Here's how the part is built. I have some questions about the finished solid (model axes, mm). A direction names the side the tool comes from. Round coordinates to 2 decimals unless told otherwise and drop trailing zeros. Loops run counter-clockwise (first coordinate to the right, second up) from the corner with the lowest first, then second, coordinate; pieces in that order, holes last. Notation, with made-up numbers: M -19.5,14.25 L 5.5,14.25 A27 ccw 5.5,38.25 Z; hole C -0.5,-40 d5. An arc over 180 degrees is marked long. Put each result on its own line as item: value. Start each with the question number.
```python
from build123d import *

# Parameters (mm, degrees)
SKETCH_1_W          = 17.5
SKETCH_1_H          = 17.5
EXTRUDE_1_DEPTH     = 8
SKETCH_2_R          = 1.35
CUT_EXTRUDE_1_DEPTH = 22.137939824
CUT_EXTRUDE_2_DEPTH = 4
SKETCH_5_W          = 6.75
SKETCH_5_H          = 17.5
EXTRUDE_3_DEPTH     = 0.2
SKETCH_6_W          = 9.75
SKETCH_6_H          = 22
EXTRUDE_4_DEPTH     = 2.5


with BuildPart() as part:
    # 草图1 → 凸台-拉伸1 (new body)
    with BuildSketch(Plane(origin=(0, 0, 0), x_dir=(1, 0, 0), z_dir=(0, 1, 0))):
        Rectangle(SKETCH_1_W, SKETCH_1_H)
    extrude(amount=EXTRUDE_1_DEPTH)

    # 草图2 → 切除-拉伸1 (cut, through all)
    with BuildSketch(Plane(origin=(8.75, 0, 0), x_dir=(0, 0, -1), z_dir=(1, 0, 0))):
        with Locations((5, 4)):
            Circle(SKETCH_2_R)
        with Locations(Location((-5, 4, 0), (0, 0, 180))):
            Circle(SKETCH_2_R)
    extrude(amount=-CUT_EXTRUDE_1_DEPTH, mode=Mode.SUBTRACT)

    # 草图3 → 切除-拉伸2 (cut)
    with BuildSketch(Plane(origin=(8.75, 0, 0), x_dir=(0, 0, -1), z_dir=(1, 0, 0))):
        Polygon((7.886751346, 4), (6.443375673, 6.5), (3.556624327, 6.5), (2.113248654, 4), (3.556624327, 1.5), (6.443375673, 1.5), align=None)
        Polygon((-6.443375673, 1.5), (-7.886751346, 4), (-6.443375673, 6.5), (-3.556624327, 6.5), (-2.113248654, 4), (-3.556624327, 1.5), align=None)
    extrude(amount=-CUT_EXTRUDE_2_DEPTH, mode=Mode.SUBTRACT)

    # 草图5 → 凸台-拉伸3 (add)
    with BuildSketch(Plane.XZ):
        with Locations((5.375, 0)):
            Rectangle(SKETCH_5_W, SKETCH_5_H)
    extrude(amount=EXTRUDE_3_DEPTH)

    # 草图6 → 凸台-拉伸4 (add)
    with BuildSketch(Plane.XZ.offset(0.2)):
        with Locations((6.875, 0)):
            Rectangle(SKETCH_6_W, SKETCH_6_H)
    extrude(amount=EXTRUDE_4_DEPTH)


solid = part.part
```
1) Suppose I cut it at C-C (y = 3.5). Write out the boundary of the cut face in (x, z), plus the area to 3 significant figures.
2) If we mould it in two halves opening along Z, with no side actions, what happens to faces 4 (the face through (0, 4, -8.75)), 5 (the face through (4.75, 5.1, -6.2)), 6 (the face through (7, -2.7, 0))? For each: pulls with the +Z half, pulls with the -Z half, needs draft (parallel to the pull), parting line crosses it, or undercut.
3) Suppose I cut it at D-D (z = -7.25). Write out the boundary of the cut face in (x, y), plus the area to 3 significant figures.
4) I'm going to push flat-ended pins straight in: P1, Ø2.5, axis at y = 3.5, z = 6, coming from the +X side; P2, Ø1.4, axis at y = -1, z = -4, coming from the -X side; P3, Ø2.5, axis at y = 4, z = 5, coming from the +X side; P4, Ø12, axis at x = -6.5, z = -1.5, coming from the -Y side. Where does each tip first touch, or does it pass through?
5) Suppose I cut it at A-A (z = -5). Write out the boundary of the cut face in (x, y).
6) On a 3-axis mill with a long thin cutter (end or side, diameter ignored), from which of +Z, -Z, +X, -X, +Y, -Y can I reach the whole of each face in a straight line? I mean faces 1 (the face through (6.778, 2.733, 7.155)), 2 (the face through (11.75, -1, 0)), 3 (the face through (2, -1, 0)). Say none if no direction works.
7) Suppose I cut it at B-B (x = -5.5). Write out the boundary of the cut face in (y, z).
8) If I drill on probe 1 along Y at (x, z) = (1.5, 5); probe 2 along Z at (x, y) = (7, 2.5); probe 3 along Z at (x, y) = (0.5, 5.5), over which ranges is the centre line in solid material (lowest first)? Write a range as from..to.
Results are:
1. outline: M -8.75,-8.75 L 8.75,-8.75 L 8.75,-7.6 L 4.75,-7.6 L 4.75,-6.25 L -8.75,-6.25 Z; M -8.75,-3.75 L 4.75,-3.75 L 4.75,-2.4 L 8.75,-2.4 L 8.75,2.4 L 4.75,2.4 L 4.75,3.75 L -8.75,3.75 Z; M -8.75,6.25 L 4.75,6.25 L 4.75,7.6 L 8.75,7.6 L 8.75,8.75 L -8.75,8.75 Z
1. area: 197 mm²
2. face 4: pulls with the -Z half
2. face 5: undercut
2. face 6: needs draft
3. outline: M -8.75,0 L 2,0 L 2,-2.7 L 11.75,-2.7 L 11.75,-0.2 L 8.75,-0.2 L 8.75,2.9 L 4.75,2.9 L 4.75,5.1 L 8.75,5.1 L 8.75,8 L -8.75,8 Z
3. area: 157 mm²
4. P1: x = 4.75
4. P2: x = 2
4. P3: through
4. P4: y = 0
5. outline: M -8.75,0 L 2,0 L 2,-2.7 L 11.75,-2.7 L 11.75,-0.2 L 8.75,-0.2 L 8.75,1.5 L 4.75,1.5 L 4.75,2.65 L -8.75,2.65 Z; M -8.75,5.35 L 4.75,5.35 L 4.75,6.5 L 8.75,6.5 L 8.75,8 L -8.75,8 Z
6. face 1: +X
6. face 2: +Z, -Z, +X, +Y, -Y
6. face 3: +Z, -Z, -X, -Y
7. outline: M 0,-8.75 L 8,-8.75 L 8,8.75 L 0,8.75 Z; hole C 4,-5 d2.7; hole C 4,5 d2.7
8. probe 1: 0..2.65, 5.35..8
8. probe 2: -8.75..-7.02, -2.98..2.98, 7.02..8.75
8. probe 3: -8.75..8.75
